Build history of the part. All positions in model axes, mm. Coordinates: 2 decimals unless noted, no trailing zeros. Order: outer loops, then holes, each group sorted by start corner. A loop starts at its lowest first (then second) coordinate and runs counter-clockwise, first axis right, second up. Notation, with made-up numbers: (-11, 88) - (32, 88) arc R28 cw to (32, 108) - close; hole circle Ø2 at (22.5, 45.5). An arc over 180 degrees is marked (long way). One line per item, written item: value.
Autodesk Inventor part; units mm, degrees
ref_plane "YZ Plane" through (0, 0, 0) normal (1, 0, 0) x (0, 1, 0)
ref_plane "XZ Plane" through (0, 0, 0) normal (0, 1, 0) x (-1, 0, 0)
ref_plane "XY Plane" through (0, 0, 0) normal (0, 0, 1) x (1, 0, 0)
sketch "Sketch1" plane through (0, 0, 0) normal (0, 0, 1) x (1, 0, 0)
  line L0 (0, 0) -> (207, 0)
  line L1 (207, 0) -> (207, 40)
  line L2 (207, 40) -> (0, 40)
  line L3 (0, 40) -> (0, 0)
  dimension "d0" = 207
  dimension "d1" = 40
extrude "Extrusion1" add sketch "Sketch1" along normal blind 5
sketch "Sketch2" plane through (0, 0, 5) normal (0, 0, 1) x (1, 0, 0)
  line L0 (207, 40) -> (0, 40)
  line L1 (0, 0) -> (207, 0)
  line L2 (0, 40) -> (0, 0)
  point P0 (17.5, 32.5)
  point P1 (17.5, 7.5)
  point P2 (112.5, 32.5)
  point P3 (112.5, 7.5)
  point P4 (186.5, 32.5)
  point P5 (186.5, 7.5)
  dimension "d4" = 7.5
  dimension "d5" = 7.5
  dimension "d6" = 17.5
  dimension "d7" = 95
  dimension "d8" = 74
hole "Hole1" at (17.5, 32.5, 5) at (17.5, 7.5, 5) at (112.5, 32.5, 5) at (112.5, 7.5, 5) at (186.5, 32.5, 5) at (186.5, 7.5, 5) direction (0, 0, -1) diameter 4.5 end through all countersink diameter 9.4 countersink angle 90
sketch "Sketch3" plane through (0, 0, 5) normal (0, 0, 1) x (1, 0, 0)
  line L0 (0, 40) -> (0, 0)
  line L1 (0, 0) -> (207, 0)
  circle A0 centre (186.5, 7.5) radius 4.7
  point P0 (159, 45)
  dimension "d17" = 45
  dimension "d25" = 27.5
hole "Hole2" at (159, 45, 5) direction (0, 0, -1) diameter 40 end through all
sketch "Sketch4" plane through (0, 0, 5) normal (0, 0, 1) x (1, 0, 0)
  line L0 (0, 0) -> (207, 0)
  line L1 (0, 40) -> (0, 0)
  point P0 (40, 10)
  point P1 (140, 10)
  dimension "d26" = 10
  dimension "d27" = 100
  dimension "d28" = 40
hole "Hole3" at (40, 10, 5) at (140, 10, 5) direction (0, 0, -1) diameter 3.4 end through all
properties part number "Top_Slider Piece 2" material "Wood (Oak)"
1. Band-saw the part on A-A, the plane x = 186.5. Give the cut face in (y, z), and give its area (3 significant figures).
Values found:
outline: (0, 0) - (5.25, 0) - (5.25, 2.55) - (2.8, 5) - (0, 5) - close; (9.75, 0) - (30.25, 0) - (30.25, 2.55) - (27.8, 5) - (12.2, 5) - (9.75, 2.55) - close; (34.75, 0) - (40, 0) - (40, 5) - (37.2, 5) - (34.75, 2.55) - close
area: 143 mm2
2. Two-plate mould, pull along Y, no slides. Class faces 1 (the face through (207, 20, 2)), 2 (the face through (193, 40, 2)), 3 (the face through (19.496, 31.462, 1.257)), 4 (the face through (102, 0, 2)): pulls with the +Y half, pulls with the -Y half, needs draft (parallel to the pull), parting line crosses it, or undercut.
Values found:
face 1: needs draft
face 2: pulls with the +Y half
face 3: undercut
face 4: pulls with the -Y half
3. Band-saw the part on D-D, the plane y = 32.5. Give the cut face in (x, z), and give its area (3 significant figures).
Values found:
outline: (0, 0) - (15.25, 0) - (15.25, 2.55) - (12.8, 5) - (0, 5) - close; (19.75, 0) - (110.25, 0) - (110.25, 2.55) - (107.8, 5) - (22.2, 5) - (19.75, 2.55) - close; (114.75, 0) - (143.39, 0) - (143.39, 5) - (117.2, 5) - (114.75, 2.55) - close; (174.61, 0) - (184.25, 0) - (184.25, 2.55) - (181.8, 5) - (174.61, 5) - close; (188.75, 0) - (207, 0) - (207, 5) - (191.2, 5) - (188.75, 2.55) - close
area: 793 mm2
4. Band-saw the part on B-B, the plane z = 4.15. Count the separate pieces of the cut face and the enclosed holes in it, and give its area (3 significant figures).
Values found:
separate pieces: 1
enclosed holes: 8
area: 7,550 mm2
5. Probe line 1 along Y through (x, z) = (186.5, 1.75); line 2 along X through (y, z) = (7.5, 0.65); line 3 along X through (y, z) = (31, 3.9). List the from-to ranges inside material, lowest first.
Values found:
line 1: y = 0 to 5.25, 9.75 to 30.25, 34.75 to 40
line 2: x = 0 to 15.25, 19.75 to 110.25, 114.75 to 184.25, 188.75 to 207
line 3: x = 0 to 14.23, 20.77 to 109.23, 115.77 to 144.72, 173.28 to 183.23, 189.77 to 207
6. Band-saw the part on C-C, the plane x = 40. Give the cut face in (y, z).
Values found:
outline: (0, 0) - (8.3, 0) - (8.3, 5) - (0, 5) - close; (11.7, 0) - (40, 0) - (40, 5) - (11.7, 5) - close
7. Flat gauge pins, fed straight in: P1, Ø2, axis at x = 40, y = 10, coming from the +Z side; P2, Ø1.5, axis at x = 163, z = 3, coming from the +Y side; P3, Ø6, axis at x = 112.5, y = 32.5, coming from the +Z side. Where does each tip first touch, or does it go through?
Values found:
P1: passes through
P2: stops at y = 25.57
P3: stops at z = 3.3
